```python
from build123d import *

# Parameters (mm, degrees)
SKETCH_1_W      = 43
SKETCH_1_H      = 60
SKETCH_1_R      = 1.5
SKETCH_1_R_2    = 2
SKETCH_1_W_2    = 20
SKETCH_1_H_2    = 42
EXTRUDE_1_DEPTH = 3


with BuildPart() as part:
    # 草图1 → 凸台-拉伸1 (new body)
    with BuildSketch(Plane(origin=(0, 0, 0), x_dir=(1, 0, 0), z_dir=(0, 1, 0))):
        with Locations((21.5, -30)):
            Rectangle(SKETCH_1_W, SKETCH_1_H)
        with Locations(Location((8, -5.7, 0), (0, 0, 270))):
            Circle(SKETCH_1_R, mode=Mode.SUBTRACT)
        with Locations(Location((18, -5.7, 0), (0, 0, 270))):
            Circle(SKETCH_1_R, mode=Mode.SUBTRACT)
        with Locations(Location((8, -54.3, 0), (0, 0, 270))):
            Circle(SKETCH_1_R, mode=Mode.SUBTRACT)
        with Locations(Location((18, -54.3, 0), (0, 0, 270))):
            Circle(SKETCH_1_R, mode=Mode.SUBTRACT)
        with Locations(Location((35, -17.5, 0), (0, 0, 270))):
            Circle(SKETCH_1_R_2, mode=Mode.SUBTRACT)
        with Locations(Location((35, -42.5, 0), (0, 0, 270))):
            Circle(SKETCH_1_R_2, mode=Mode.SUBTRACT)
        with Locations((13, -30)):
            Rectangle(SKETCH_1_W_2, SKETCH_1_H_2, mode=Mode.SUBTRACT)
    extrude(amount=EXTRUDE_1_DEPTH)


solid = part.part
```
The model under review builds one solid part; all positions refer to its coordinate system, in mm. A direction names the side the tool comes from. Give positions to 0.01 mm unless a question says otherwise; leave off trailing zeros. Order: outer loops, then holes, each group sorted by start corner. A loop starts at its lowest first (then second) coordinate and runs counter-clockwise, first axis right, second up. Notation, with made-up numbers: (3, 87) - (37, 87) arc R32 cw to (37, 126) - close; hole circle Ø6 at (67.25, 38). An arc over 180 degrees is marked (long way). Use CSV: the item, a comma, the result in double quotes. Start each with the question number.
Q1. To check wall thickness, follow line 1 along X through (y, z) = (1.3, 5.7); line 2 along X through (y, z) = (2.1, 17.5); line 3 along X through (y, z) = (0.75, 36). State the ranges of each line that lie inside material, in increasing order. Write a range as [from, to].
Q2. We need section D-D, the plane y = 1.8. Write out the cut boundary in (x, z), and give its area (3 significant figures).
Q3. We need section B-B, the plane z = 33. Write out the cut boundary in (x, y).
Q4. Clearance check with a flat-ended pin moving along its axis: pin 1 Ø12 at (x, z) = (10, 17.5) entering from -Y. State where the tip first meets the part, or that it passes through.
Q5. Tool access review of faces 5 (the flat face through (21, 1, 0)), 6 (the flat face through (3, 1, 30)): name each direction out of +Z, -Z, +X, -X, +Y, -Y from which nothing blocks a thin tool from reaching the whole face with its end or side.
Q6. We need section C-C, the plane x = 35. Write out the cut boundary in (y, z).
Q7. The part is to be moulded in two halves that separate along X. For faces 1 (the cylindrical face through (19.265, 1.479, 55.106)), 2 (the flat face through (26, 3, 30)), 3 (the flat face through (43, 1, 30)), 4 (the flat face through (0, 1, 30)), say which applies: +X half, -X half, draft (parallel to the pull), parting line (faces both ways), or undercut.
Q8. We need section A-A, the plane x = 11.5. Write out the cut boundary in (y, z).
Outcome:
1,line 1,"x = [0, 6.5], [9.5, 16.5], [19.5, 43]"
1,line 2,"x = [0, 3], [23, 33], [37, 43]"
1,line 3,"x = [0, 3], [23, 43]"
2,outline,"(0, 0) - (43, 0) - (43, 60) - (0, 60) - close; hole (3, 9) - (23, 9) - (23, 51) - (3, 51) - close; hole circle Ø3 at (8, 5.7); hole circle Ø3 at (8, 54.3); hole circle Ø3 at (18, 5.7); hole circle Ø3 at (18, 54.3); hole circle Ø4 at (35, 17.5); hole circle Ø4 at (35, 42.5)"
2,area,"1,690 mm^2"
3,outline,"(0, 0) - (3, 0) - (3, 3) - (0, 3) - close; (23, 0) - (43, 0) - (43, 3) - (23, 3) - close"
4,pin 1,"passes through"
5,face 5,"-Z, +X, -X, +Y, -Y"
5,face 6,"+Y, -Y"
6,outline,"(0, 0) - (3, 0) - (3, 15.5) - (0, 15.5) - close; (0, 19.5) - (3, 19.5) - (3, 40.5) - (0, 40.5) - close; (0, 44.5) - (3, 44.5) - (3, 60) - (0, 60) - close"
7,face 1,"undercut"
7,face 2,"draft"
7,face 3,"+X half"
7,face 4,"-X half"
8,outline,"(0, 0) - (3, 0) - (3, 9) - (0, 9) - close; (0, 51) - (3, 51) - (3, 60) - (0, 60) - close"
